Can you work these out from the model? Positions are in its coordinate system, mm. Face numbers are marked on the shaded views. Round coordinates to 2 decimals unless told otherwise and drop trailing zeros. Order: outer loops, then holes, each group sorted by start corner. A loop starts at its lowest first (then second) coordinate and runs counter-clockwise, first axis right, second up.
Q1. If we section it at D-D (y = 80.5): Please give me the cut outline in (x, z), plus the area to 3 significant figures.
Q2. If we section it at B-B (z = -42.5): Please give me the cut outline in (x, y).
Q3. If I drill on line 1 (Y direction, x = 3, z = -54); line 2 (Z direction, x = 6, y = 5.25); line 3 (Z direction, x = 7, y = 203.5), over which ranges is the centre line in solid material (lowest first)?
Q4. If we section it at A-A (y = 140): Please give me the cut outline in (x, z).
Q5. If we section it at C-C (y = 20): Please give me the cut outline in (x, z).
Q6. Will these pins go through, and if not, where does the flat tip stop? P1, Ø5.5, axis at x = 6, z = -12.5, coming from the -Y side; P2, Ø6.5, axis at y = 20, z = -42.5, coming from the +X side; P3, Ø1, axis at x = 7, y = 198, coming from the +Z side; P4, Ø1.5, axis at x = 10.5, z = -32, coming from the +Y side.
Q7. We'd pull the mould along Z, two halves only. Please class the marked faces 1, 2, 3 and 4: pulls with the +Z half, pulls with the -Z half, needs draft (parallel to the pull), parting line crosses it, or undercut.
from build123d import *

# Parameters (mm, degrees)
BOSS_EXTRUDE1_DEPTH = 12
CUT_EXTRUDE1_REACH  = 270.596
SKETCH2_R           = 4
CUT_EXTRUDE2_REACH  = 270.596
SKETCH3_R           = 3
CUT_EXTRUDE3_REACH  = 270.596
SKETCH4_R           = 13
SKETCH4_R_2         = 6
SKETCH4_R_3         = 2
CUT_EXTRUDE4_REACH  = 270.596
SKETCH5_R           = 3


with BuildPart() as part:
    # Sketch1 → Boss-Extrude1 (new body)
    with BuildSketch(Plane(origin=(0, 0, 0), x_dir=(0, 0, -1), z_dir=(1, 0, 0))):
        Polygon((120, 240), (35, 240), (35, 120), (0, 38), (0, 0), (85, 0), (85, 38), (120, 120), align=None)
    extrude(amount=BOSS_EXTRUDE1_DEPTH)

    # Sketch2 → Cut-Extrude1 (cut, up to next)
    with BuildSketch(Plane.ZY, mode=Mode.PRIVATE) as cut_extrude1_sk1:
        with Locations((-42.5, 20)):
            Circle(SKETCH2_R)
    cut_extrude1_tool1 = extrude(cut_extrude1_sk1.sketch, amount=-CUT_EXTRUDE1_REACH, mode=Mode.PRIVATE) & part.part
    # Sketch2 → Cut-Extrude1 (cut, up to next)
    with BuildSketch(Plane.ZY, mode=Mode.PRIVATE) as cut_extrude1_sk2:
        with Locations((-72.5, 20)):
            Circle(SKETCH2_R)
    cut_extrude1_tool2 = extrude(cut_extrude1_sk2.sketch, amount=-CUT_EXTRUDE1_REACH, mode=Mode.PRIVATE) & part.part
    # Sketch2 → Cut-Extrude1 (cut, up to next)
    with BuildSketch(Plane.ZY, mode=Mode.PRIVATE) as cut_extrude1_sk3:
        with Locations((-12.5, 20)):
            Circle(SKETCH2_R)
    cut_extrude1_tool3 = extrude(cut_extrude1_sk3.sketch, amount=-CUT_EXTRUDE1_REACH, mode=Mode.PRIVATE) & part.part
    add(cut_extrude1_tool1.solids().sort_by_distance((0, 20, -42.5))[0], mode=Mode.SUBTRACT)
    add(cut_extrude1_tool2.solids().sort_by_distance((0, 20, -72.5))[0], mode=Mode.SUBTRACT)
    add(cut_extrude1_tool3.solids().sort_by_distance((0, 20, -12.5))[0], mode=Mode.SUBTRACT)

    # Sketch3 → Cut-Extrude2 (cut, up to next)
    with BuildSketch(Plane.XZ, mode=Mode.PRIVATE) as cut_extrude2_sk1:
        with Locations(Location((6, -42.5, 0), (0, 0, 270))):
            Circle(SKETCH3_R)
    cut_extrude2_tool1 = extrude(cut_extrude2_sk1.sketch, amount=-CUT_EXTRUDE2_REACH, mode=Mode.PRIVATE) & part.part
    # Sketch3 → Cut-Extrude2 (cut, up to next)
    with BuildSketch(Plane.XZ, mode=Mode.PRIVATE) as cut_extrude2_sk2:
        with Locations(Location((6, -72.5, 0), (0, 0, 270))):
            Circle(SKETCH3_R)
    cut_extrude2_tool2 = extrude(cut_extrude2_sk2.sketch, amount=-CUT_EXTRUDE2_REACH, mode=Mode.PRIVATE) & part.part
    # Sketch3 → Cut-Extrude2 (cut, up to next)
    with BuildSketch(Plane.XZ, mode=Mode.PRIVATE) as cut_extrude2_sk3:
        with Locations(Location((6, -12.5, 0), (0, 0, 270))):
            Circle(SKETCH3_R)
    cut_extrude2_tool3 = extrude(cut_extrude2_sk3.sketch, amount=-CUT_EXTRUDE2_REACH, mode=Mode.PRIVATE) & part.part
    add(cut_extrude2_tool1.solids().sort_by_distance((6, 0, -42.5))[0], mode=Mode.SUBTRACT)
    add(cut_extrude2_tool2.solids().sort_by_distance((6, 0, -72.5))[0], mode=Mode.SUBTRACT)
    add(cut_extrude2_tool3.solids().sort_by_distance((6, 0, -12.5))[0], mode=Mode.SUBTRACT)

    # Sketch4 → Cut-Extrude3 (cut, up to next)
    with BuildSketch(Plane.ZY, mode=Mode.PRIVATE) as cut_extrude3_sk1:
        with Locations((-77.5, 180)):
            Circle(SKETCH4_R)
    cut_extrude3_tool1 = extrude(cut_extrude3_sk1.sketch, amount=-CUT_EXTRUDE3_REACH, mode=Mode.PRIVATE) & part.part
    # Sketch4 → Cut-Extrude3 (cut, up to next)
    with BuildSketch(Plane.ZY, mode=Mode.PRIVATE) as cut_extrude3_sk2:
        with Locations((-77.5, 220)):
            Circle(SKETCH4_R_2)
    cut_extrude3_tool2 = extrude(cut_extrude3_sk2.sketch, amount=-CUT_EXTRUDE3_REACH, mode=Mode.PRIVATE) & part.part
    # Sketch4 → Cut-Extrude3 (cut, up to next)
    with BuildSketch(Plane.ZY, mode=Mode.PRIVATE) as cut_extrude3_sk3:
        with Locations((-77.5, 140)):
            Circle(SKETCH4_R_2)
    cut_extrude3_tool3 = extrude(cut_extrude3_sk3.sketch, amount=-CUT_EXTRUDE3_REACH, mode=Mode.PRIVATE) & part.part
    # Sketch4 → Cut-Extrude3 (cut, up to next)
    with BuildSketch(Plane.ZY, mode=Mode.PRIVATE) as cut_extrude3_sk4:
        with Locations((-101, 203.5)):
            Circle(SKETCH4_R_3)
    cut_extrude3_tool4 = extrude(cut_extrude3_sk4.sketch, amount=-CUT_EXTRUDE3_REACH, mode=Mode.PRIVATE) & part.part
    # Sketch4 → Cut-Extrude3 (cut, up to next)
    with BuildSketch(Plane.ZY, mode=Mode.PRIVATE) as cut_extrude3_sk5:
        with Locations((-54, 203.5)):
            Circle(SKETCH4_R_3)
    cut_extrude3_tool5 = extrude(cut_extrude3_sk5.sketch, amount=-CUT_EXTRUDE3_REACH, mode=Mode.PRIVATE) & part.part
    # Sketch4 → Cut-Extrude3 (cut, up to next)
    with BuildSketch(Plane.ZY, mode=Mode.PRIVATE) as cut_extrude3_sk6:
        with Locations((-101, 156.5)):
            Circle(SKETCH4_R_3)
    cut_extrude3_tool6 = extrude(cut_extrude3_sk6.sketch, amount=-CUT_EXTRUDE3_REACH, mode=Mode.PRIVATE) & part.part
    # Sketch4 → Cut-Extrude3 (cut, up to next)
    with BuildSketch(Plane.ZY, mode=Mode.PRIVATE) as cut_extrude3_sk7:
        with Locations((-54, 156.5)):
            Circle(SKETCH4_R_3)
    cut_extrude3_tool7 = extrude(cut_extrude3_sk7.sketch, amount=-CUT_EXTRUDE3_REACH, mode=Mode.PRIVATE) & part.part
    add(cut_extrude3_tool1.solids().sort_by_distance((0, 180, -77.5))[0], mode=Mode.SUBTRACT)
    add(cut_extrude3_tool2.solids().sort_by_distance((0, 220, -77.5))[0], mode=Mode.SUBTRACT)
    add(cut_extrude3_tool3.solids().sort_by_distance((0, 140, -77.5))[0], mode=Mode.SUBTRACT)
    add(cut_extrude3_tool4.solids().sort_by_distance((0, 203.5, -101))[0], mode=Mode.SUBTRACT)
    add(cut_extrude3_tool5.solids().sort_by_distance((0, 203.5, -54))[0], mode=Mode.SUBTRACT)
    add(cut_extrude3_tool6.solids().sort_by_distance((0, 156.5, -101))[0], mode=Mode.SUBTRACT)
    add(cut_extrude3_tool7.solids().sort_by_distance((0, 156.5, -54))[0], mode=Mode.SUBTRACT)

    # Sketch5 → Cut-Extrude4 (cut, up to next)
    with BuildSketch(Plane.ZY, mode=Mode.PRIVATE) as cut_extrude4_sk1:
        with Locations((-114, 210)):
            Circle(SKETCH5_R)
    cut_extrude4_tool1 = extrude(cut_extrude4_sk1.sketch, amount=-CUT_EXTRUDE4_REACH, mode=Mode.PRIVATE) & part.part
    # Sketch5 → Cut-Extrude4 (cut, up to next)
    with BuildSketch(Plane.ZY, mode=Mode.PRIVATE) as cut_extrude4_sk2:
        with Locations((-114, 150)):
            Circle(SKETCH5_R)
    cut_extrude4_tool2 = extrude(cut_extrude4_sk2.sketch, amount=-CUT_EXTRUDE4_REACH, mode=Mode.PRIVATE) & part.part
    add(cut_extrude4_tool1.solids().sort_by_distance((0, 210, -114))[0], mode=Mode.SUBTRACT)
    add(cut_extrude4_tool2.solids().sort_by_distance((0, 150, -114))[0], mode=Mode.SUBTRACT)


solid = part.part
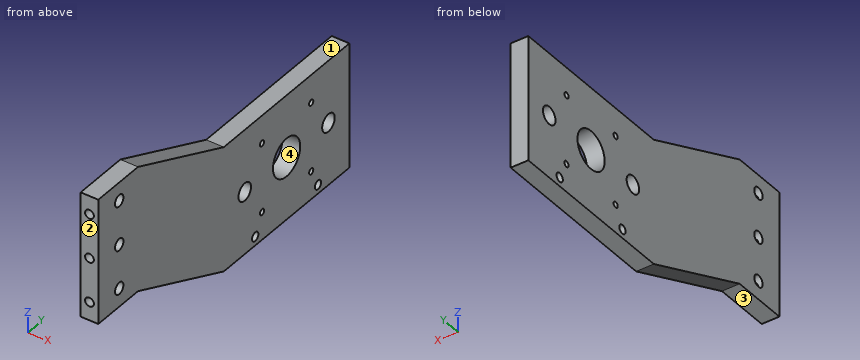
Solution:
1. outline: (0, -103.14) - (12, -103.14) - (12, -18.14) - (0, -18.14) - close
1. area: 1,020 mm2
2. outline: (0, 0) - (3, 0) - (3, 16) - (0, 16) - close; (0, 24) - (12, 24) - (12, 240) - (0, 240) - close; (9, 0) - (12, 0) - (12, 16) - (9, 16) - close
3. line 1: y = 0 to 154.5, 158.5 to 201.5, 205.5 to 240
3. line 2: z = -85 to -75.5, -69.5 to -45.5, -39.5 to -15.5, -9.5 to 0
3. line 3: z = -120 to -103, -99 to -56, -52 to -35
4. outline: (0, -120) - (12, -120) - (12, -83.5) - (0, -83.5) - close; (0, -71.5) - (12, -71.5) - (12, -35) - (0, -35) - close
5. outline: (0, -85) - (12, -85) - (12, -76.5) - (0, -76.5) - close; (0, -68.5) - (12, -68.5) - (12, -46.5) - (0, -46.5) - close; (0, -38.5) - (12, -38.5) - (12, -16.5) - (0, -16.5) - close; (0, -8.5) - (12, -8.5) - (12, 0) - (0, 0) - close
6. P1: stops at y = 22.9
6. P2: passes through
6. P3: stops at z = -35
6. P4: stops at y = 114.73
7. face 1: pulls with the +Z half
7. face 2: needs draft
7. face 3: pulls with the -Z half
7. face 4: undercut
